Design review of the part built by this model. Coordinates are the model's own, in mm. A direction names the side the tool comes from. Coordinates: 2 decimals unless noted, no trailing zeros. Loops run counter-clockwise (first coordinate to the right, second up) from the corner with the lowest first, then second, coordinate; pieces in that order, holes last. Notation, with made-up numbers: (8, -3) -> (59, -3) arc R7 cw to (59, 6) -> close; hole circle Ø1 at (3.5, 86.5). An arc over 180 degrees is marked (long way). Answer in a Markdown table with one row per item.
```python
from build123d import *

# Parameters (mm, degrees)
SKETCH1_W           = 38.1
SKETCH1_H           = 63.5
BOSS_EXTRUDE1_DEPTH = 9
SKETCH1_3_W         = 10
SKETCH1_3_H         = 30.48
BOSS_EXTRUDE2_DEPTH = 40
SKETCH2_R           = 1.5
CUT_EXTRUDE1_DEPTH  = 10
SKETCH3_R           = 1.375
BOSS_EXTRUDE3_DEPTH = 10
CUT_EXTRUDE2_DEPTH  = 9


with BuildPart() as part:
    # Sketch1 → Boss-Extrude1 (new body)
    with BuildSketch(Plane(origin=(0, 0, 0), x_dir=(1, 0, 0), z_dir=(0, 1, 0))):
        Rectangle(SKETCH1_W, SKETCH1_H)
    extrude(amount=BOSS_EXTRUDE1_DEPTH)

    # Sketch1<3> → Boss-Extrude2 (add)
    with BuildSketch(Plane(origin=(0, 0, 0), x_dir=(1, 0, 0), z_dir=(0, 1, 0))):
        with Locations((-24.05, -16.51)):
            Rectangle(SKETCH1_3_W, SKETCH1_3_H)
    extrude(amount=BOSS_EXTRUDE2_DEPTH)

    # Sketch2 → Cut-Extrude1 (cut)
    with BuildSketch(Plane.ZY.offset(29.05)):
        with Locations((4.55, 19.7)):
            Circle(SKETCH2_R)
        with Locations((26.75, 30)):
            Circle(SKETCH2_R)
    extrude(amount=-CUT_EXTRUDE1_DEPTH, mode=Mode.SUBTRACT)

    # Sketch3 → Boss-Extrude3 (add)
    with BuildSketch(Plane(origin=(0, 0, -31.75), x_dir=(-1, 0, 0), z_dir=(0, 0, -1))):
        Polygon((-19.05, 0), (19.05, 0), (19.05, 50), (8.05, 50), (8.05, 30), (-1.95, 30), (-1.95, 50), (-19.05, 50), align=None)
        with Locations((-6.95, 25)):
            Circle(SKETCH3_R, mode=Mode.SUBTRACT)
        with Locations((-6.95, 45)):
            Circle(SKETCH3_R, mode=Mode.SUBTRACT)
        with Locations((13.05, 25)):
            Circle(SKETCH3_R, mode=Mode.SUBTRACT)
        with Locations((13.05, 45)):
            Circle(SKETCH3_R, mode=Mode.SUBTRACT)
    extrude(amount=BOSS_EXTRUDE3_DEPTH)

    # Sketch1<4> → Cut-Extrude2 (cut)
    with BuildSketch(Plane(origin=(0, 0, 0), x_dir=(1, 0, 0), z_dir=(0, 1, 0))):
        with BuildLine():
            ThreePointArc((4.064, -6.35), (2.873681959, -3.476318041), (0, -2.286))
            Line((0, -2.286), (0, -10.414))
            ThreePointArc((0, -10.414), (2.873681959, -9.223681959), (4.064, -6.35))
        make_face()
        with BuildLine():
            Line((0, -10.414), (0, -2.286))
            ThreePointArc((0, -2.286), (-4.064, -6.35), (0, -10.414))
        make_face()
    extrude(amount=CUT_EXTRUDE2_DEPTH, mode=Mode.SUBTRACT)


solid = part.part
```
(1) Draft analysis for pull direction Y (two halves, no side actions). For faces 4 (the cylindrical face through (-24.12, 20.71, 3.44)), 5 (the flat face through (-19.05, 14, -34)), 6 (the cylindrical face through (6.32, 43.78, -36.68)), 7 (the flat face through (-14, 50, -37)), state which applies: pulls with the +Y half, pulls with the -Y half, needs draft (parallel to the pull), parting line crosses it, or undercut.
Evaluation:
| item | result |
|---|---|
| face 4 | undercut |
| face 5 | needs draft |
| face 6 | undercut |
| face 7 | pulls with the +Y half |
(2) Take a section at C-C on y = 13. Give the boundary of the cut face in (x, z).
Evaluation:
| item | result |
|---|---|
| outline | (-29.05, 1.27) -> (-19.05, 1.27) -> (-19.05, 31.75) -> (-29.05, 31.75) -> close; (-19.05, -41.75) -> (19.05, -41.75) -> (19.05, -31.75) -> (-19.05, -31.75) -> close |
(3) Take a section at A-A on x = -13.05. Give the boundary of the cut face in (y, z) (3 decimals).
Evaluation:
| item | result |
|---|---|
| outline | (0, -41.75) -> (23.625, -41.75) -> (23.625, -31.75) -> (9, -31.75) -> (9, 31.75) -> (0, 31.75) -> close; (26.375, -41.75) -> (43.625, -41.75) -> (43.625, -31.75) -> (26.375, -31.75) -> close; (46.375, -41.75) -> (50, -41.75) -> (50, -31.75) -> (46.375, -31.75) -> close |
(4) Take a section at D-D on z = -33. Give the boundary of the cut face in (x, y) (3 decimals).
Evaluation:
| item | result |
|---|---|
| outline | (-19.05, 0) -> (19.05, 0) -> (19.05, 50) -> (1.95, 50) -> (1.95, 30) -> (-8.05, 30) -> (-8.05, 50) -> (-19.05, 50) -> close; hole circle Ø2.75 at (-13.05, 25); hole circle Ø2.75 at (-13.05, 45); hole circle Ø2.75 at (6.95, 25); hole circle Ø2.75 at (6.95, 45) |
(5) Tool access review of faces 1 (the flat face through (-24, 20, 1.27)), 2 (the flat face through (0, 9, 0)), 3 (the flat face through (0.3, 29.8, -31.75)): name each direction out of +Z, -Z, +X, -X, +Y, -Y from which nothing blocks a thin tool from reaching the whole face with its end or side.
Evaluation:
| item | result |
|---|---|
| face 1 | -Z, -X, +Y, -Y |
| face 2 | +Z, +X, +Y |
| face 3 | +Z, +X, -X, +Y |
(6) To check wall thickness, follow probe 1 along Y at (x, z) = (6.95, -34.25) (3 decimals); probe 2 along Y at (x, z) = (6, -37); probe 3 along Y at (x, z) = (-16, -1). State the ranges of each line that lie inside material, in increasing order.
Evaluation:
| item | result |
|---|---|
| probe 1 | y = 0 to 23.625, 26.375 to 43.625, 46.375 to 50 |
| probe 2 | y = 0 to 24.01, 25.99 to 44.01, 45.99 to 50 |
| probe 3 | y = 0 to 9 |
(7) Take a section at B-B on y = 25. Give the boundary of the cut face in (x, z) (3 decimals).
Evaluation:
| item | result |
|---|---|
| outline | (-29.05, 1.27) -> (-19.05, 1.27) -> (-19.05, 31.75) -> (-29.05, 31.75) -> close; (-19.05, -41.75) -> (-14.425, -41.75) -> (-14.425, -31.75) -> (-19.05, -31.75) -> close; (-11.675, -41.75) -> (5.575, -41.75) -> (5.575, -31.75) -> (-11.675, -31.75) -> close; (8.325, -41.75) -> (19.05, -41.75) -> (19.05, -31.75) -> (8.325, -31.75) -> close |
(8) For pin 1 (3 mm diameter, centred on x = -23.5, z = 21.5, fed in from +Y); pin 2 (4.5 mm diameter, centred on x = -13.05, y = 45, fed in from +Z); pin 3 (5 mm diameter, centred on y = 44.5, z = -36.5, fed in from -X); pin 4 (5 mm diameter, centred on y = 30, z = 26.75, fed in from -X), all flat-tipped, find the tip position at first contact; note any pin that passes through.
Evaluation:
| item | result |
|---|---|
| pin 1 | stops at y = 40 |
| pin 2 | stops at z = -31.75 |
| pin 3 | stops at x = -19.05 |
| pin 4 | stops at x = -29.05 |
